```python
from build123d import *

# Parameters (mm, degrees)
SKETCH_1_R               = 5
EXTRUDE_1_DEPTH          = 1
SKETCH_1_6_R             = 0.5
CUT_EXTRUDE_2_DEPTH      = 8.141428429
SKETCH_1_7_R             = 0.6
CUT_EXTRUDE_3_DEPTH      = 2
PATTERN_CIRCULAR_1_COUNT = 4


with BuildPart() as part:
    # Sketch 1 → Extrude 1 (new body)
    with BuildSketch(Plane(origin=(0, 0, 0), x_dir=(1, 0, 0), z_dir=(0, 1, 0))):
        with Locations(Location((0, 0, 0), (0, 0, 270))):
            Circle(SKETCH_1_R)
    extrude(amount=EXTRUDE_1_DEPTH)

    # Sketch 1_6 → Cut-Extrude 2 (cut, through all)
    with BuildSketch(Plane(origin=(0, 0, 0), x_dir=(1, 0, 0), z_dir=(0, 1, 0))):
        with Locations(Location((0, 0, 0), (0, 0, 270))):
            Circle(SKETCH_1_6_R)
    extrude(amount=CUT_EXTRUDE_2_DEPTH, mode=Mode.SUBTRACT)

    # Sketch 1_7 → Cut-Extrude 3 (cut)
    with BuildSketch(Plane(origin=(0, 0, 0), x_dir=(1, 0, 0), z_dir=(0, 1, 0))):
        with Locations(Location((-3.875, 0, 0), (0, 0, 270))):
            Circle(SKETCH_1_7_R)
    cut_extrude_3 = extrude(amount=CUT_EXTRUDE_3_DEPTH, mode=Mode.SUBTRACT)

    # Pattern Circular 1: Cut-Extrude 3 ×4 about axis
    pattern_circular_1_axis = Axis((0, 0, 0), (0, 1, 0))
    for i in range(1, PATTERN_CIRCULAR_1_COUNT):
        add(cut_extrude_3.rotate(pattern_circular_1_axis, i * 360 / PATTERN_CIRCULAR_1_COUNT), mode=Mode.SUBTRACT)


solid = part.part
```
Work out the finished part from the listing and answer in its coordinate system (mm). Coordinates: 2 decimals unless noted, no trailing zeros. Loops run counter-clockwise (first coordinate to the right, second up) from the corner with the lowest first, then second, coordinate; pieces in that order, holes last. Notation, with made-up numbers: (88.5, 68.5) -> (93.5, 68.5) arc R12 ccw to (93.5, 74.5) -> close; hole circle Ø11 at (-14.75, 39). An arc over 180 degrees is marked (long way). Answer as CSV lines item,"result".
Q1. The part is cut by section B-B on x = 0. Write down the section's boundary in (y, z) (3 decimals), and give its area (3 significant figures).
Findings:
outline,"(0, -5) -> (1, -5) -> (1, -4.475) -> (0, -4.475) -> close; (0, -3.275) -> (1, -3.275) -> (1, -0.5) -> (0, -0.5) -> close; (0, 0.5) -> (1, 0.5) -> (1, 3.275) -> (0, 3.275) -> close; (0, 4.475) -> (1, 4.475) -> (1, 5) -> (0, 5) -> close"
area,"6.60 mm²"
Q2. The part is cut by section D-D on x = 3.75. Write down the section's boundary in (y, z), and give its area (3 significant figures).
Findings:
outline,"(0, -3.31) -> (1, -3.31) -> (1, -0.59) -> (0, -0.59) -> close; (0, 0.59) -> (1, 0.59) -> (1, 3.31) -> (0, 3.31) -> close"
area,"5.44 mm²"
Q3. Find the intervals of material crossed by probe 1 along X at (y, z) = (0.4, 0) (3 decimals); probe 2 along X at (y, z) = (0.9, 3.75); probe 3 along X at (y, z) = (0.2, -3.5), in increasing order.
Findings:
probe 1,"x = -5 to -4.475, -3.275 to -0.5, 0.5 to 3.275, 4.475 to 5"
probe 2,"x = -3.31 to -0.59, 0.59 to 3.31"
probe 3,"x = -3.57 to -0.47, 0.47 to 3.57"
Q4. The part is cut by section C-C on y = 0.5. Write down the section's boundary in (x, z) (3 decimals), and give its area (3 significant figures).
Findings:
outline,"circle Ø10 at (0, 0); hole circle Ø1.2 at (-3.875, 0); hole circle Ø1.2 at (0, -3.875); hole circle Ø1.2 at (0, 3.875); hole circle Ø1 at (0, 0); hole circle Ø1.2 at (3.875, 0)"
area,"73.2 mm²"
Q5. For a pull along Z with two mould halves and no side action, classify faces 1 (the face through (-0.08, 0.49, 3.28)), 2 (the face through (0.08, 0.49, -3.28)), 3 (the face through (-1, 1, 0)), 4 (the face through (-4.88, 0.49, -1.08)) as +Z half, -Z half, draft (parallel to the pull), parting line (faces both ways), or undercut.
Findings:
face 1,"undercut"
face 2,"undercut"
face 3,"draft"
face 4,"parting line"
Q6. This flat-tipped pin is pushed along its axis until it touches: pin 1 (1.1 mm diameter, centred on x = 0, z = -3.875, fed in from -Y). Where does it stop, or does it pass through?
Findings:
pin 1,"passes through"
Q7. The part is cut by section A-A on z = 0. Write down the section's boundary in (x, y) (3 decimals).
Findings:
outline,"(-5, 0) -> (-4.475, 0) -> (-4.475, 1) -> (-5, 1) -> close; (-3.275, 0) -> (-0.5, 0) -> (-0.5, 1) -> (-3.275, 1) -> close; (0.5, 0) -> (3.275, 0) -> (3.275, 1) -> (0.5, 1) -> close; (4.475, 0) -> (5, 0) -> (5, 1) -> (4.475, 1) -> close"
